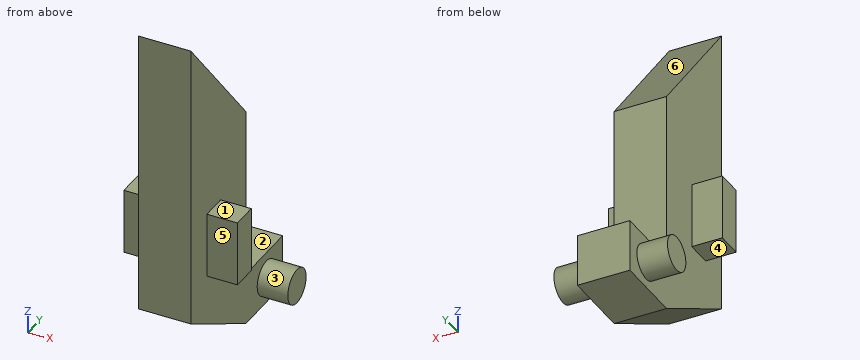
from build123d import *

# Parameters (mm, degrees)
SKETCH1_W           = 12
SKETCH1_H           = 24
BOSS_EXTRUDE1_DEPTH = 80
CUT_EXTRUDE1_DEPTH  = 12
SKETCH4_W           = 15
SKETCH4_H           = 6
BOSS_EXTRUDE2_DEPTH = 7
SKETCH5_W           = 12
SKETCH5_H           = 12
BOSS_EXTRUDE3_DEPTH = 16
SKETCH7_R           = 4
BOSS_EXTRUDE4_DEPTH = 13


with BuildPart() as part:
    # Sketch1 → Boss-Extrude1 (new body)
    with BuildSketch(Plane.XY):
        with Locations((0, 12)):
            Rectangle(SKETCH1_W, SKETCH1_H)
    extrude(amount=-BOSS_EXTRUDE1_DEPTH)

    # Sketch2 → Cut-Extrude1 (cut)
    with BuildSketch(Plane(origin=(6, 0, 0), x_dir=(0, 0, -1), z_dir=(1, 0, 0))):
        Polygon((0, 24), (0, 0), (28.602086222, 24), align=None)
        Polygon((80, 24), (66.143593539, 0), (80, 0), align=None)
    extrude(amount=-CUT_EXTRUDE1_DEPTH, mode=Mode.SUBTRACT)

    # Sketch4 → Boss-Extrude2 (add)
    with BuildSketch(Plane(origin=(6, 0, 0), x_dir=(0, 0, -1), z_dir=(1, 0, 0))):
        with Locations((51.102086222, 10)):
            Rectangle(SKETCH4_W, SKETCH4_H)
    boss_extrude2 = extrude(amount=BOSS_EXTRUDE2_DEPTH)

    # Mirror1: Boss-Extrude2 across plane
    add(boss_extrude2.mirror(Plane(origin=(0, 0, 0), x_dir=(0, 0, 1), z_dir=(1, 0, 0))))

    # Sketch5 → Boss-Extrude3 (add)
    with BuildSketch(Plane(origin=(0, 24, 0), x_dir=(1, 0, 0), z_dir=(0, 1, 0))):
        with Locations((0, 74)):
            Rectangle(SKETCH5_W, SKETCH5_H)
    extrude(amount=BOSS_EXTRUDE3_DEPTH)

    # Sketch7 → Boss-Extrude4 (add, symmetric)
    with BuildSketch(Plane(origin=(0, 0, 0), x_dir=(0, 0, -1), z_dir=(1, 0, 0))):
        with Locations((74, 32.938039716)):
            Circle(SKETCH7_R)
    extrude(amount=BOSS_EXTRUDE4_DEPTH, both=True)


solid = part.part
Geometry: final body of the model. Coordinates: model frame, mm. Face numbers are marked on the shaded views. A direction names the side the tool comes from. Coordinates: 2 decimals unless noted, no trailing zeros. Loops run counter-clockwise (first coordinate to the right, second up) from the corner with the lowest first, then second, coordinate; pieces in that order, holes last. Notation, with made-up numbers: M 17.5,60 L 40.5,60 A22 ccw 40.5,79 Z; hole C 33,-22.75 d5. An arc over 180 degrees is marked long. One line per item, written item: value. Start each with the question number.
1) Cut plane B-B (x = 2.25). Return loops of the section in (y, z).
2) Cut plane C-C (y = 30.5). Return loops of the section in (x, z).
3) Draft query along Z for the marked faces 4, 5 and 6. Return one class per face: released by +Z, released by -Z, zero draft, split by the parting line, or undercut.
4) Cut plane A-A (z = -57). Return loops of the section in (x, y).
5) Cut plane D-D (x = -6.75). Return loops of the section in (y, z).
6) Material intervals for L1, parallel to Z at x = 8.5, y = 11; L2, parallel to X at y = 23.5, z = -50; L3, parallel to Y at x = -0.25, z = -29, sorted ascending. Write a range as from..to.
7) Pin query (flat end, axial travel): P1, Ø1, axis at y = 8, z = -61.5, coming from the +X side; P2, Ø3, axis at x = 11, y = 10.5, coming from the -Z side; P3, Ø1, axis at x = -6, z = -59, coming from the +Y side; P4, Ø1, axis at x = 7.5, z = -59.5, coming from the +Y side. Return the tip coordinate at first contact, or that it passes through.
8) Reachability of the marked faces 1, 2 and 3 from +Z, -Z, +X, -X, +Y, -Y: full face, straight path, thin tool, end or side. Return the list, or none.
Evaluation:
1. outline: M 0,-66.14 L 24,-80 L 40,-80 L 40,-68 L 24,-68 L 24,-28.6 L 0,0 Z
2. outline: M -13,-77.17 L -6,-77.17 L -6,-80 L 6,-80 L 6,-77.17 L 13,-77.17 L 13,-70.83 L 6,-70.83 L 6,-68 L -6,-68 L -6,-70.83 L -13,-70.83 Z
3. face 4: released by -Z
3. face 5: zero draft
3. face 6: released by +Z
4. outline: M -13,7 L -6,7 L -6,0 L 6,0 L 6,7 L 13,7 L 13,13 L 6,13 L 6,24 L -6,24 L -6,13 L -13,13 Z
5. outline: M 7,-58.6 L 13,-58.6 L 13,-43.6 L 7,-43.6 Z; C 32.94,-74 d8
6. L1: -58.6..-43.6
6. L2: -6..6
6. L3: 0..24
7. P1: x = 6
7. P2: z = -58.6
7. P3: y = 24
7. P4: through
8. face 1: +Z, +X, +Y, -Y
8. face 2: +Z, +X, -X, +Y
8. face 3: +X
